Source: CAD feature listing. Evaluate the final solid. Frame: model axes, mm. Face numbers are marked on the shaded views. A direction names the side the tool comes from. Round coordinates to 2 decimals unless told otherwise and drop trailing zeros. Loops run counter-clockwise (first coordinate to the right, second up) from the corner with the lowest first, then second, coordinate; pieces in that order, holes last. Notation, with made-up numbers: M -12,10.5 L 17,10.5 A17 ccw 17,36.5 Z; hole C 71,56 d1. An arc over 180 degrees is marked long. Answer as a JSON object with one key per item and string values.
from build123d import *

# Parameters (mm, degrees)
BASPROSKE_W        = 5.5
BASPROSKE_H        = 9.2
TOOTHCUT_DEPTH     = 15.12550884
TEETHCUTS_COUNT    = 21
TEETHCUTS_ANGLE    = 342.857142857
BORSKE_R           = 1
BORE_DEPTH         = 50.0000508
SKETCH1_R          = 1
CUT_EXTRUDE1_DEPTH = 5.5


with BuildPart() as part:
    # BasProSke → Base-Revolve (revolve)
    with BuildSketch(Plane(origin=(0, 0, 0), x_dir=(1, 0, 0), z_dir=(0, 1, 0)), mode=Mode.PRIVATE) as base_revolve_sk:
        with Locations((2.75, 4.6)):
            Rectangle(BASPROSKE_W, BASPROSKE_H)
    revolve(base_revolve_sk.sketch.rotate(Axis((-10, 0, 0), (1, 0, 0)), 180), axis=Axis((-10, 0, 0), (1, 0, 0)))

    # TooCutSke → ToothCut (cut, through all)
    with BuildSketch(Plane(origin=(0, 0, 0), x_dir=(0, 0, -1), z_dir=(1, 0, 0))):
        with BuildLine():
            ThreePointArc((0.39557227, 7.388418205), (0, 7.399), (-0.39557227, 7.388418205))
            ThreePointArc((-0.39557227, 7.388418205), (-0.659317872, 8.326513344), (-1.181161837, 9.149473311))
            ThreePointArc((-1.181161837, 9.149473311), (0, 9.2254), (1.181161837, 9.149473311))
            ThreePointArc((1.181161837, 9.149473311), (0.659317872, 8.326513344), (0.39557227, 7.388418205))
        make_face()
    toothcut = extrude(amount=TOOTHCUT_DEPTH, mode=Mode.SUBTRACT)

    # TeethCuts: ToothCut ×21 about axis
    teethcuts_axis = Axis((-10, 0, 0), (1, 0, 0))
    for i in range(1, TEETHCUTS_COUNT):
        add(toothcut.rotate(teethcuts_axis, i * TEETHCUTS_ANGLE / (TEETHCUTS_COUNT - 1)), mode=Mode.SUBTRACT)

    # BorSke → Bore (cut, symmetric)
    with BuildSketch(Plane(origin=(0, 0, 0), x_dir=(0, 0, -1), z_dir=(1, 0, 0))):
        with Locations(Location((0, 0, 0), (0, 0, 180))):
            Circle(BORSKE_R)
    extrude(amount=BORE_DEPTH, both=True, mode=Mode.SUBTRACT)

    # Sketch1 → Cut-Extrude1 (cut)
    with BuildSketch(Plane(origin=(5.5, 0, 0), x_dir=(0, 0, -1), z_dir=(1, 0, 0))):
        with Locations((2.121320344, -2.121320344)):
            Circle(SKETCH1_R)
    extrude(amount=-CUT_EXTRUDE1_DEPTH, mode=Mode.SUBTRACT)


solid = part.part
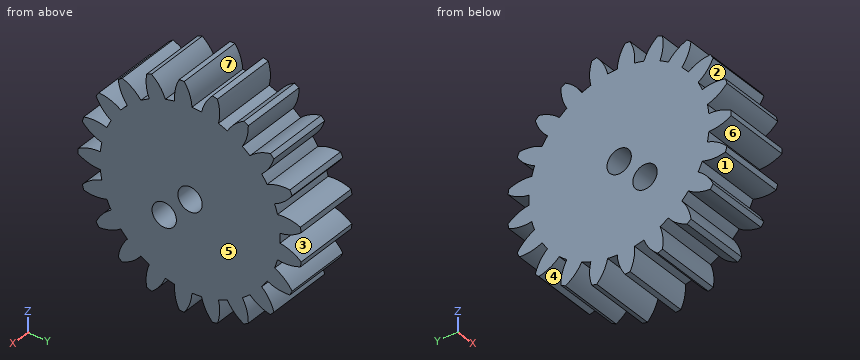
Item 1: Section B-B on x = 1.6. Give the number of separate pieces and of enclosed holes in the cut face, then the cut area to 3 significant figures.
Answer sheet:
{"separate pieces": "1", "enclosed holes": "2", "area": "208 mm²"}
Item 2: Section C-C on y = 5.5. Return the cut outline in (x, z).
Answer sheet:
{"outline": "M 0,-5.98 L 5.5,-5.98 L 5.5,5.98 L 0,5.98 Z"}
Item 3: Pull-direction query (Z, two-part tool) for the marked faces 4, 5, 6 and 7; classes: pulls with the +Z half, pulls with the -Z half, needs draft (parallel to the pull), parting line crosses it, or undercut.
Answer sheet:
{"face 4": "pulls with the -Z half", "face 5": "needs draft", "face 6": "undercut", "face 7": "pulls with the +Z half"}
Item 4: Access query for the marked faces 1, 2 and 3. Directions: +Z, -Z, +X, -X, +Y, -Y. A direction counts if a zero-diameter tool reaches every point of the face in a straight line with its end or side. Return the directions, or none.
Answer sheet:
{"face 1": "+X, -X", "face 2": "+X, -X, -Y", "face 3": "+X, -X, +Y"}
Item 5: Section A-A on y = -2.75. Return the cut outline in (x, z).
Answer sheet:
{"outline": "M 0,-8.27 L 5.5,-8.27 L 5.5,-2.9 L 0,-2.9 Z; M 0,-1.34 L 5.5,-1.34 L 5.5,8.27 L 0,8.27 Z"}
Item 6: Contact query for a flat-ended pin moving along its axis: pin 1 Ø1.6 at (y, z) = (0, 0) entering from +X. Output: stop coordinate, or through.
Answer sheet:
{"pin 1": "passes through"}
Item 7: Line query: probe 1 along Z at (x, y) = (3.9, 6.5); probe 2 along Y at (x, z) = (3.65, -8); probe 3 along Y at (x, z) = (3, 8.25). Output: solid intervals per line, ascending. Write a range as from..to.
Answer sheet:
{"probe 1": "z = -6.39..-5.22, -3.92..3.92, 5.22..6.39", "probe 2": "y = -3.61..-2.52, -1.25..0.07, 1.16..2.43, 4.29..4.54", "probe 3": "y = -3.59..-2.73, -1.21..0, 1.28..2.41"}
